Read the model definition and answer for the solid it produces. Units are mm, in the model's axes. A direction names the side the tool comes from. Give positions to 0.01 mm unless a question says otherwise; leave off trailing zeros. Loops run counter-clockwise (first coordinate to the right, second up) from the corner with the lowest first, then second, coordinate; pieces in that order, holes last. Notation, with made-up numbers: (44, -13.5) - (81, -13.5) arc R17 ccw to (81, 0.5) - close; hole circle Ø1 at (40, 74). An arc over 180 degrees is marked (long way). Use a Markdown table: item, result. Add a question column.
Item 1: A cutting plane is placed at D-D (x = 57). Determine the outline of the cut face in (y, z).
Item 2: Which of the six approach directions +Z, -Z, +X, -X, +Y, -Y give full straight-line access (tool end or side, diameter ignored) to faces 1 (the face through (50, 36.5, 2)), 2 (the face through (46, 15, 2)), 3 (the face through (27, -7.2, 4.2)), 4 (the face through (19, -7, 2)), 5 (the face through (0.162, -5.255, 4.909))?
Item 3: Each of these flat-tipped pins is pushed along its axis until it touches: P1, Ø1.2, axis at y = 31, z = 1.5, coming from the +X side; P2, Ø3, axis at x = 57, y = -13.5, coming from the +Z side; P3, Ø2, axis at x = 16, z = 2.5, coming from the +Y side. Where does it stop, or does it pass through?
Item 4: A cutting plane is placed at C-C (y = 30). Determine the outline of the cut face in (x, z), plus the area to 3 significant figures.
Item 5: For a pull along X with two mould halves and no side action, classify faces 6 (the face through (62.4, 32, 2)), 7 (the face through (-13, 0, 2)), 8 (the face through (34, 11, 2)), 9 (the face through (-3, 3, 8)) as +X half, -X half, draft (parallel to the pull), parting line (faces both ways), or undercut.
Item 6: A cutting plane is placed at B-B (x = 46.5). Determine the outline of the cut face in (y, z).
Item 7: Consider probe 1 along X at (y, z) = (30, 0.95); probe 2 along Y at (x, z) = (44.5, 3.75); probe 3 along Y at (x, z) = (57, 1.5). Determine where each line is inside the solid, lowest interval first. Write a range as [from, to].
Item 8: A cutting plane is placed at A-A (z = 5). Determine the outline of the cut face in (x, y), plus the area to 3 significant figures.
from build123d import *

# Parameters (mm, degrees)
ELBOW_HORN_FLANGE_PROFILE_R          = 13
ELBOW_HORN_FLANGE_DEPTH              = 4
FOREARM_WEB_PROFILE_W                = 40
FOREARM_WEB_PROFILE_H                = 14
FOREARM_WEB_DEPTH                    = 4
GRIPPER_MOUNT_RIB_PROFILE_W          = 8
GRIPPER_MOUNT_RIB_PROFILE_H          = 30
GRIPPER_MOUNT_RIB_DEPTH              = 4
GRIPPER_SERVO_MOUNT_PROFILE_W        = 44
GRIPPER_SERVO_MOUNT_PROFILE_H        = 26
GRIPPER_SERVO_MOUNT_DEPTH            = 4
GRIP_SG90_BODY_CLEARANCE_START       = -5
GRIP_SG90_BODY_CLEARANCE_PROFILE_W   = 23.8
GRIP_SG90_BODY_CLEARANCE_PROFILE_H   = 13
GRIP_SG90_BODY_CLEARANCE_DEPTH       = 87.221918224
MOVING_FINGER_SWEEP_RELIEF_START     = -5
MOVING_FINGER_SWEEP_RELIEF_PROFILE_W = 13
MOVING_FINGER_SWEEP_RELIEF_PROFILE_H = 13
MOVING_FINGER_SWEEP_RELIEF_DEPTH     = 87.221918224
GRIP_SERVO_TAB_FASTENERS_START       = -50
GRIP_SERVO_TAB_FASTENERS_PROFILE_R   = 1.3
GRIP_SERVO_TAB_FASTENERS_DEPTH       = 132.221918224
FIXED_FINGER_SPINE_PROFILE_W         = 48
FIXED_FINGER_SPINE_PROFILE_H         = 5
FIXED_FINGER_SPINE_DEPTH             = 4
FIXED_FINGER_ROOT_PROFILE_W          = 7
FIXED_FINGER_ROOT_PROFILE_H          = 23
FIXED_FINGER_ROOT_DEPTH              = 7
ELBOW_CENTER_SCREW_ACCESS_START      = -50
ELBOW_CENTER_SCREW_ACCESS_PROFILE_R  = 4
ELBOW_CENTER_SCREW_ACCESS_DEPTH      = 139.396832522
ELBOW_DOWEL_SUPPORT_HUB_START        = 4
ELBOW_DOWEL_SUPPORT_HUB_PROFILE_R    = 7
ELBOW_DOWEL_SUPPORT_HUB_PROFILE_R_2  = 4
ELBOW_DOWEL_SUPPORT_HUB_DEPTH        = 4
ELBOW_HORN_FASTENERS_START           = -50
ELBOW_HORN_FASTENERS_PROFILE_R       = 1.1
ELBOW_HORN_FASTENERS_DEPTH           = 139.481636513
M2X8_WASHER_AND_HUB_CLEARANCE_START  = 3
ELBOW_HORN_WASHER_RECESS_PROFILE_R   = 2.75
M2X8_WASHER_AND_HUB_CLEARANCE_DEPTH  = 5
FIXED_PAD_KEEPER_FASTENERS_START     = -50
FIXED_PAD_KEEPER_FASTENERS_PROFILE_R = 1.1
FIXED_PAD_KEEPER_FASTENERS_DEPTH     = 139.481636513


with BuildPart() as part:
    # Elbow_horn_flange_profile → Elbow_horn_flange (new body)
    with BuildSketch(Plane.XY):
        Circle(ELBOW_HORN_FLANGE_PROFILE_R)
    extrude(amount=ELBOW_HORN_FLANGE_DEPTH)

    # Forearm_web_profile → Forearm_web (add)
    with BuildSketch(Plane.XY):
        with Locations((20, 0)):
            Rectangle(FOREARM_WEB_PROFILE_W, FOREARM_WEB_PROFILE_H)
    extrude(amount=FOREARM_WEB_DEPTH)

    # Gripper_mount_rib_profile → Gripper_mount_rib (add)
    with BuildSketch(Plane.XY):
        with Locations((30, 15)):
            Rectangle(GRIPPER_MOUNT_RIB_PROFILE_W, GRIPPER_MOUNT_RIB_PROFILE_H)
    extrude(amount=GRIPPER_MOUNT_RIB_DEPTH)

    # Gripper_servo_mount_profile → Gripper_servo_mount (add)
    with BuildSketch(Plane.XY):
        with Locations((48, 28)):
            Rectangle(GRIPPER_SERVO_MOUNT_PROFILE_W, GRIPPER_SERVO_MOUNT_PROFILE_H)
    extrude(amount=GRIPPER_SERVO_MOUNT_DEPTH)

    # Grip_SG90_body_clearance_profile → Grip_SG90_body_clearance (cut, through all)
    with BuildSketch(Plane.XY.offset(GRIP_SG90_BODY_CLEARANCE_START)):
        with Locations((50.5, 30)):
            Rectangle(GRIP_SG90_BODY_CLEARANCE_PROFILE_W, GRIP_SG90_BODY_CLEARANCE_PROFILE_H)
    extrude(amount=GRIP_SG90_BODY_CLEARANCE_DEPTH, mode=Mode.SUBTRACT)

    # Moving_finger_sweep_relief_profile → Moving_finger_sweep_relief (cut, through all)
    with BuildSketch(Plane.XY.offset(MOVING_FINGER_SWEEP_RELIEF_START)):
        with Locations((64.5, 20.5)):
            Rectangle(MOVING_FINGER_SWEEP_RELIEF_PROFILE_W, MOVING_FINGER_SWEEP_RELIEF_PROFILE_H)
    extrude(amount=MOVING_FINGER_SWEEP_RELIEF_DEPTH, mode=Mode.SUBTRACT)

    # Grip_servo_tab_fasteners_profile → Grip_servo_tab_fasteners (cut, through all)
    with BuildSketch(Plane.XY.offset(GRIP_SERVO_TAB_FASTENERS_START)):
        with Locations((36, 30)):
            Circle(GRIP_SERVO_TAB_FASTENERS_PROFILE_R)
        with Locations((65, 30)):
            Circle(GRIP_SERVO_TAB_FASTENERS_PROFILE_R)
    extrude(amount=GRIP_SERVO_TAB_FASTENERS_DEPTH, mode=Mode.SUBTRACT)



with BuildPart() as body_2:
    # Fixed_finger_spine_profile → Fixed_finger_spine (new body)
    with BuildSketch(Plane.XY):
        with Locations((54, -13.5)):
            Rectangle(FIXED_FINGER_SPINE_PROFILE_W, FIXED_FINGER_SPINE_PROFILE_H)
    extrude(amount=FIXED_FINGER_SPINE_DEPTH)


with BuildPart() as part_1:
    add(part.part)

    add(body_2.part)  # Fixed_finger_root merges body 2
    # Fixed_finger_root_profile → Fixed_finger_root (add)
    with BuildSketch(Plane.XY):
        with Locations((30.5, -4.5)):
            Rectangle(FIXED_FINGER_ROOT_PROFILE_W, FIXED_FINGER_ROOT_PROFILE_H)
    extrude(amount=FIXED_FINGER_ROOT_DEPTH)

    # Elbow_center_screw_access_profile → Elbow_center_screw_access (cut, through all)
    with BuildSketch(Plane.XY.offset(ELBOW_CENTER_SCREW_ACCESS_START)):
        with Locations(Location((0, 0, 0), (0, 0, 180))):
            Circle(ELBOW_CENTER_SCREW_ACCESS_PROFILE_R)
    extrude(amount=ELBOW_CENTER_SCREW_ACCESS_DEPTH, mode=Mode.SUBTRACT)

    # Elbow_dowel_support_hub_profile → Elbow_dowel_support_hub (add)
    with BuildSketch(Plane.XY.offset(ELBOW_DOWEL_SUPPORT_HUB_START)):
        Circle(ELBOW_DOWEL_SUPPORT_HUB_PROFILE_R)
        with Locations(Location((0, 0, 0), (0, 0, 180))):
            Circle(ELBOW_DOWEL_SUPPORT_HUB_PROFILE_R_2, mode=Mode.SUBTRACT)
    extrude(amount=ELBOW_DOWEL_SUPPORT_HUB_DEPTH)

    # Elbow_horn_fasteners_profile → Elbow_horn_fasteners (cut, through all)
    with BuildSketch(Plane.XY.offset(ELBOW_HORN_FASTENERS_START)):
        with Locations(Location((0, -8, 0), (0, 0, 112.9239414))):
            Circle(ELBOW_HORN_FASTENERS_PROFILE_R)
        with Locations(Location((0, 8, 0), (0, 0, 247.0760586))):
            Circle(ELBOW_HORN_FASTENERS_PROFILE_R)
        with Locations(Location((-8, 0, 0), (0, 0, 22.9239414))):
            Circle(ELBOW_HORN_FASTENERS_PROFILE_R)
        with Locations(Location((8, 0, 0), (0, 0, 157.0760586))):
            Circle(ELBOW_HORN_FASTENERS_PROFILE_R)
    extrude(amount=ELBOW_HORN_FASTENERS_DEPTH, mode=Mode.SUBTRACT)

    # Elbow_horn_washer_recess_profile → M2x8_washer_and_hub_clearance (cut)
    with BuildSketch(Plane.XY.offset(M2X8_WASHER_AND_HUB_CLEARANCE_START)):
        with Locations(Location((0, -8, 0), (0, 0, 149.150544772))):
            Circle(ELBOW_HORN_WASHER_RECESS_PROFILE_R)
        with Locations(Location((0, 8, 0), (0, 0, 210.849455228))):
            Circle(ELBOW_HORN_WASHER_RECESS_PROFILE_R)
        with Locations(Location((-8, 0, 0), (0, 0, 59.150544772))):
            Circle(ELBOW_HORN_WASHER_RECESS_PROFILE_R)
        with Locations(Location((8, 0, 0), (0, 0, 120.849455228))):
            Circle(ELBOW_HORN_WASHER_RECESS_PROFILE_R)
    extrude(amount=M2X8_WASHER_AND_HUB_CLEARANCE_DEPTH, mode=Mode.SUBTRACT)

    # Fixed_pad_keeper_fasteners_profile → Fixed_pad_keeper_fasteners (cut, through all)
    with BuildSketch(Plane.XY.offset(FIXED_PAD_KEEPER_FASTENERS_START)):
        with Locations(Location((57, -13.5, 0), (0, 0, 180))):
            Circle(FIXED_PAD_KEEPER_FASTENERS_PROFILE_R)
        with Locations(Location((73, -13.5, 0), (0, 0, 180))):
            Circle(FIXED_PAD_KEEPER_FASTENERS_PROFILE_R)
    extrude(amount=FIXED_PAD_KEEPER_FASTENERS_DEPTH, mode=Mode.SUBTRACT)


solid = part_1.part
Geometry says:
| question | item | result |
|---|---|---|
| 1 | outline | (-16, 0) - (-14.6, 0) - (-14.6, 4) - (-16, 4) - close; (-12.4, 0) - (-11, 0) - (-11, 4) - (-12.4, 4) - close; (15, 0) - (23.5, 0) - (23.5, 4) - (15, 4) - close; (36.5, 0) - (41, 0) - (41, 4) - (36.5, 4) - close |
| 2 | face 1 | +Z, -Z |
| 2 | face 2 | +Z, -Z, +X |
| 2 | face 3 | +Z, -Y |
| 2 | face 4 | +Z, -Z, -Y |
| 2 | face 5 | +Z |
| 3 | P1 | x = 70 |
| 3 | P2 | z = 4 |
| 3 | P3 | y = 7 |
| 4 | outline | (26, 0) - (34.7, 0) - (34.7, 4) - (26, 4) - close; (37.3, 0) - (38.6, 0) - (38.6, 4) - (37.3, 4) - close; (62.4, 0) - (63.7, 0) - (63.7, 4) - (62.4, 4) - close; (66.3, 0) - (70, 0) - (70, 4) - (66.3, 4) - close |
| 4 | area | 60.0 mm² |
| 5 | face 6 | undercut |
| 5 | face 7 | undercut |
| 5 | face 8 | +X half |
| 5 | face 9 | draft |
| 6 | outline | (-16, 0) - (-11, 0) - (-11, 4) - (-16, 4) - close; (15, 0) - (23.5, 0) - (23.5, 4) - (15, 4) - close; (36.5, 0) - (41, 0) - (41, 4) - (36.5, 4) - close |
| 7 | probe 1 | [26, 34.7], [37.3, 38.6], [62.4, 63.7], [66.3, 70] |
| 7 | probe 2 | [-16, -11], [15, 23.5], [36.5, 41] |
| 7 | probe 3 | [-16, -14.6], [-12.4, -11], [15, 23.5], [36.5, 41] |
| 8 | outline | (-6.59, -2.36) arc R7 ccw to (-2.36, -6.59) arc R2.75 cw to (2.36, -6.59) arc R7 ccw to (6.59, -2.36) arc R2.75 cw to (6.59, 2.36) arc R7 ccw to (2.36, 6.59) arc R2.75 cw to (-2.36, 6.59) arc R7 ccw to (-6.59, 2.36) arc R2.75 cw to start; (27, -16) - (34, -16) - (34, 7) - (27, 7) - close; hole circle Ø8 at (0, 0) |
| 8 | area | 242 mm² |
